Build history of the part. All positions in model axes, mm. Give positions to 0.01 mm unless a question says otherwise; leave off trailing zeros. Order: outer loops, then holes, each group sorted by start corner. A loop starts at its lowest first (then second) coordinate and runs counter-clockwise, first axis right, second up. Notation, with made-up numbers: (58.5, 24.25) - (82.5, 24.25) arc R4 cw to (82.5, 30.25) - close; hole circle Ø11 at (2, 41). An arc over 180 degrees is marked (long way). Use a Markdown table: item, result. Add a question column.
(1) Wall check: line 1 (Y direction, x = 175.5, z = 4.6); line 2 (X direction, y = 349.5, z = 0.95); line 3 (X direction, y = 237.5, z = 4.65). Give the ranges that are in metal, low to high.
(2) Slice it at A-A (z = 3.9). Write the cut outline in (x, y), then the cut area to 3 significant figures.
(3) Slice it at C-C (x = 108.5). Write the cut outline in (y, z), then the cut area to 4 significant figures.
(4) Slice it at B-B (y = 294.5). Write the cut outline in (x, z), then the cut area to 3 significant figures.
(5) Flat gauge pins, fed straight in: pin 1 (3 mm diameter, centred on y = 77.5, z = 4, fed in from +X); pin 2 (2.5 mm diameter, centred on y = 342.5, z = 3.5, fed in from -X); pin 3 (1.5 mm diameter, centred on x = 82.5, z = 2.5, fed in from -Y). Where does each tip first touch, or does it go through?
from build123d import *

# Parameters (mm, degrees)
SKETCH1_W           = 120
SKETCH1_H           = 137.6
SKETCH1_W_2         = 200
SKETCH1_H_2         = 160
BOSS_EXTRUDE1_DEPTH = 5
CHAMFER1_SIZE       = 70
CHAMFER2_SIZE       = 40


with BuildPart() as part:
    # Sketch1 → Boss-Extrude1 (new body)
    with BuildSketch(Plane.XY):
        with Locations((0, 323.8)):
            Rectangle(SKETCH1_W, SKETCH1_H)
        with Locations((-160, 175)):
            Rectangle(SKETCH1_W_2, SKETCH1_H_2)
        with Locations((0, 175)):
            Rectangle(SKETCH1_W, SKETCH1_H_2)
        with Locations((160, 175)):
            Rectangle(SKETCH1_W_2, SKETCH1_H_2)
        with Locations((0, 26.2)):
            Rectangle(SKETCH1_W, SKETCH1_H)
    extrude(amount=BOSS_EXTRUDE1_DEPTH)

    # Chamfer1
    chamfer1_edges = [part.edges().sort_by_distance(p)[0] for p in [
        (60, 255, 2.5),
        (60, 95, 2.5),
        (-60, 95, 2.5),
        (-60, 255, 2.5),
    ]]
    chamfer(chamfer1_edges, length=CHAMFER1_SIZE)

    # Chamfer2
    chamfer2_edges = [part.edges().sort_by_distance(p)[0] for p in [
        (260, 255, 2.5),
        (260, 95, 2.5),
        (-260, 95, 2.5),
        (-260, 255, 2.5),
    ]]
    chamfer(chamfer2_edges, length=CHAMFER2_SIZE)


solid = part.part
Solution:
| question | item | result |
|---|---|---|
| 1 | line 1 | 95 to 255 |
| 1 | line 2 | -60 to 60 |
| 1 | line 3 | -237.5 to 237.5 |
| 2 | outline | (-260, 135) - (-220, 95) - (-130, 95) - (-60, 25) - (-60, -42.6) - (60, -42.6) - (60, 25) - (130, 95) - (220, 95) - (260, 135) - (260, 215) - (220, 255) - (130, 255) - (60, 325) - (60, 392.6) - (-60, 392.6) - (-60, 325) - (-130, 255) - (-220, 255) - (-260, 215) - close |
| 2 | area | 123,000 mm2 |
| 3 | outline | (73.5, 0) - (276.5, 0) - (276.5, 5) - (73.5, 5) - close |
| 3 | area | 1,015 mm2 |
| 4 | outline | (-90.5, 0) - (90.5, 0) - (90.5, 5) - (-90.5, 5) - close |
| 4 | area | 905 mm2 |
| 5 | pin 1 | x = 114 |
| 5 | pin 2 | x = -60 |
| 5 | pin 3 | y = 46.75 |
